The listing builds one solid part. Answer for the finished solid, in the listing's coordinates (mm). Face numbers are marked on the shaded views. Coordinates: 2 decimals unless noted, no trailing zeros. Write each loop counter-clockwise with the first axis right and the second up, starting at its lowest first coordinate (ties: lowest second). Pieces come first, ordered by that corner, then holes.
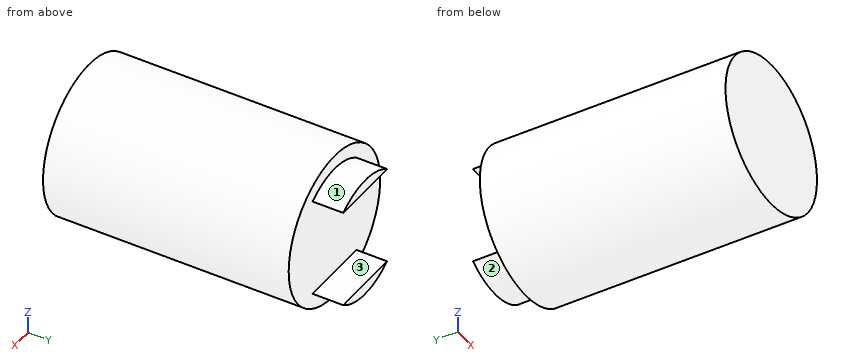
from build123d import *

# Parameters (mm, degrees)
SKETCH1_R           = 31.115
BOSS_EXTRUDE4_DEPTH = 101.6
BOSS_EXTRUDE6_DEPTH = 12.7


with BuildPart() as part:
    # Sketch1 → Boss-Extrude4 (new body)
    with BuildSketch(Plane(origin=(0, 0, 0), x_dir=(1, 0, 0), z_dir=(0, 1, 0))):
        Circle(SKETCH1_R)
    extrude(amount=BOSS_EXTRUDE4_DEPTH)

    # Sketch4 → Boss-Extrude6 (add)
    with BuildSketch(Plane(origin=(0, 101.6, 0), x_dir=(1, 0, 0), z_dir=(0, 1, 0))):
        with BuildLine():
            ThreePointArc((14.859, 20.600245605), (0, 25.4), (-14.859, 20.600245605))
            Line((-14.859, 20.600245605), (14.859, 20.600245605))
        make_face()
        with BuildLine():
            Line((14.859, -20.600245605), (-14.859, -20.600245605))
            ThreePointArc((-14.859, -20.600245605), (0, -25.4), (14.859, -20.600245605))
        make_face()
    extrude(amount=BOSS_EXTRUDE6_DEPTH)


solid = part.part
1. Section D-D on y = 58 is taken. Give the vertices of the cut face in (x, z) (3 decimals), then the cut area to 3 significant figures.
Results found:
outline: circle Ø62.23 at (0, 0)
area: 3,040 mm2
2. Section A-A on y = 107.5 is taken. Give the vertices of the cut face in (x, z).
Results found:
outline: (-14.86, -20.6) arc R25.4 ccw to (14.86, -20.6) - close; (-14.86, 20.6) - (14.86, 20.6) arc R25.4 ccw to start
3. Section B-B on x = 0 is taken. Give the vertices of the cut face in (y, z) (3 decimals).
Results found:
outline: (0, -31.115) - (101.6, -31.115) - (101.6, -25.4) - (114.3, -25.4) - (114.3, -20.6) - (101.6, -20.6) - (101.6, 20.6) - (114.3, 20.6) - (114.3, 25.4) - (101.6, 25.4) - (101.6, 31.115) - (0, 31.115) - close
4. Section C-C on z = 0 is taken. Give the vertices of the cut face in (x, y) (3 decimals), then the cut area to 3 significant figures.
Results found:
outline: (-31.115, 0) - (31.115, 0) - (31.115, 101.6) - (-31.115, 101.6) - close
area: 6,320 mm2
5. Flat-ended cylindrical pins translate along their axes: P1, Ø3, axis at x = 10, z = -0.5, coming from the +Y side; P2, Ø1, axis at y = 82, z = 24.5, coming from the +X side; P3, Ø10, axis at x = -15, y = 98.5, coming from the -Z side. Find the tip coordinate at first contact, or state that the pin passes through.
Results found:
P1: stops at y = 101.6
P2: stops at x = 19.8
P3: stops at z = -29.46
6. Find the intervals of material crossed by L1, parallel to Y at x = -12, z = -25; L2, parallel to X at y = 95, z = -0.5; L3, parallel to Z at x = -9, y = 45, in increasing order.
Results found:
L1: y = 0 to 101.6
L2: x = -31.11 to 31.11
L3: z = -29.78 to 29.78
7. For a pull along Z with two mould halves and no side action, classify the marked faces 1, 2 and 3 as pulls with the +Z half, pulls with the -Z half, needs draft (parallel to the pull), parting line crosses it, or undercut.
Results found:
face 1: pulls with the +Z half
face 2: pulls with the -Z half
face 3: undercut
